```python
from build123d import *

# Parameters (mm, degrees)
AUFSATZ_LINEAR_AUSTRAGEN1_DEPTH      = 10
SKIZZE2_W                            = 60
SKIZZE2_H                            = 10
AUFSATZ_LINEAR_AUSTRAGEN2_DEPTH      = 10
SCHNITT_LINEAR_AUSTRAGEN2_DEPTH      = 7.5
SCHNITT_LINEAR_AUSTRAGEN2_DEPTH_BACK = 7.5
FASE1_SIZE                           = 2
VERRUNDUNG1_R                        = 3


with BuildPart() as part:
    # Skizze1 → Aufsatz-Linear austragen1 (new body)
    with BuildSketch(Plane.XY):
        Polygon((40, 10), (0, 60), (0, 0), (60, 0), (60, 10), align=None)
    extrude(amount=AUFSATZ_LINEAR_AUSTRAGEN1_DEPTH)

    # Skizze2 → Aufsatz-Linear austragen2 (add)
    with BuildSketch(Plane(origin=(0, 0, 0), x_dir=(-1, 0, 0), z_dir=(0, 0, -1))):
        with Locations((-30, 5)):
            Rectangle(SKIZZE2_W, SKIZZE2_H)
    extrude(amount=AUFSATZ_LINEAR_AUSTRAGEN2_DEPTH)

    # Skizze4 → Schnitt-Linear austragen2 (cut, two sides: drawn at the far end of the back side and taken through both)
    with BuildSketch(Plane.XY.offset(-SCHNITT_LINEAR_AUSTRAGEN2_DEPTH_BACK)):
        Polygon((60, 10), (45, 10), (45, 2), (58, 2), (58, 5), (60, 5), align=None)
    extrude(amount=SCHNITT_LINEAR_AUSTRAGEN2_DEPTH + SCHNITT_LINEAR_AUSTRAGEN2_DEPTH_BACK, mode=Mode.SUBTRACT)

    # Fase1
    fase1_edges = [part.edges().sort_by_distance(p)[0] for p in [
        (58, 5, 0),
    ]]
    chamfer(fase1_edges, length=FASE1_SIZE - 0.0001)  # a hair under: the kernel refuses the full size

    # Verrundung1
    verrundung1_edges = [part.edges().sort_by_distance(p)[0] for p in [
        (45, 6, -7.5),
        (45, 6, 7.5),
    ]]
    fillet(verrundung1_edges, radius=VERRUNDUNG1_R)


solid = part.part
```
Part model, mm, in its own coordinate system. A direction names the side the tool comes from. Give positions to 0.01 mm unless a question says otherwise; leave off trailing zeros. Order: outer loops, then holes, each group sorted by start corner. A loop starts at its lowest first (then second) coordinate and runs counter-clockwise, first axis right, second up. Notation, with made-up numbers: (61.5, 55) - (105.5, 55) arc R12 ccw to (105.5, 77) - close; hole circle Ø2 at (14, 36). An arc over 180 degrees is marked (long way). Use one line per item in the form item = value.
Item 1: Probe probe 1 along Y at (x, z) = (36.5, -5); probe 2 along Y at (x, z) = (49, 2.75). List the from-to ranges inside material, lowest first. Write a range as from..to.
Solution:
probe_1 = 0..10
probe_2 = 0..2
Item 2: Slice it at A-A on x = 26. Give the cut face in (y, z).
Solution:
outline = (0, -10) - (10, -10) - (10, 0) - (27.5, 0) - (27.5, 10) - (0, 10) - close
Item 3: Two-plate mould, pull along X, no slides. Class faces 1 (the face through (0, 23, 2)), 2 (the face through (59, 4, 0)), 3 (the face through (16, 17, 10)): released by +X, released by -X, zero draft, split by the parting line, or undercut.
Solution:
face_1 = released by -X
face_2 = undercut
face_3 = zero draft
Item 4: Which spindle directions (+Z, -Z, +X, -X, +Y, -Y) get a long thin tool onto all of the face, cutting with end or side? Do faces 4 (the face through (11, 24, 0)), 5 (the face through (30, 10, -4)), 6 (the face through (30, 0, 0)), 7 (the face through (20, 35, 5)), 8 (the face through (45.86, 5.94, -6.6)). Say none if no direction does.
Solution:
face_4 = -Z, +X, -X, +Y
face_5 = -Z, +X, +Y
face_6 = +Z, -Z, +X, -X, -Y
face_7 = +Z, -Z, +X, +Y
face_8 = +Y
Item 5: Pin check, flat tips, straight feed: pin 1 Ø6 at (x, y) = (18, 26.5) entering from -Z; pin 2 Ø10.5 at (x, z) = (54, -2) entering from +Y; pin 3 Ø1 at (y, z) = (42.5, 4.5) entering from +X. Stop position of each tip, or through.
Solution:
pin_1 = 0
pin_2 = 4.25
pin_3 = 14.4
Item 6: Slice it at C-C on y = 49. Give the cut face in (x, z), and give its area (3 significant figures).
Solution:
outline = (0, 0) - (8.8, 0) - (8.8, 10) - (0, 10) - close
area = 88.0 mm2
Item 7: Slice it at D-D on x = 38. Give the cut face in (y, z), and give its area (3 significant figures).
Solution:
outline = (0, -10) - (10, -10) - (10, 0) - (12.5, 0) - (12.5, 10) - (0, 10) - close
area = 225 mm2
